CAD build for the part. Positions are in the model's coordinates, mm. Face numbers are marked on the shaded views. Give positions to 0.01 mm unless a question says otherwise; leave off trailing zeros. Use one line per item in the form item = value.
```python
from build123d import *

# Parameters (mm, degrees)
F0_W      = 40
F0_H      = 40
F1_DEPTH  = 10
F3_DEPTH  = 30
F4_R      = 5
F6_R      = 32.5
F7_DEPTH  = 5
F9_ANGLE  = -225
F10_ANGLE = -35.264


with BuildPart() as f1:
    # F0 (on Top) → F1 (new body)
    with BuildSketch(Plane.XY):
        with Locations((20, 20)):
            Rectangle(F0_W, F0_H)
    extrude(amount=F1_DEPTH)

    # F2 (on face) → F3 (join)
    with BuildSketch(Plane.XY.offset(10)):
        Polygon((0, 40), (0, 0), (40, 0), (40, 10), (10, 10), (10, 40), align=None)
    extrude(amount=F3_DEPTH)

    # F4
    f4_edges = [f1.edges().sort_by_distance(p)[0] for p in [
        (20, 0, 40),
        (0, 20, 40),
        (0, 0, 20),
        (20, 0, 0),
        (0, 20, 0),
        (20, 40, 0),
        (40, 20, 0),
        (40, 0, 20),
        (0, 40, 20),
    ]]
    fillet(f4_edges, radius=F4_R)

    # F6 (on 3pt) → F7 (cut)
    with BuildSketch(Plane(origin=(30, 30, 30), x_dir=(-0.8164965809, 0.4082482905, 0.4082482905), z_dir=(0.5773502692, 0.5773502692, 0.5773502692))):
        Circle(F6_R)
    extrude(amount=-F7_DEPTH, mode=Mode.SUBTRACT)


with BuildPart() as f1_1:
    # F9: moved
    add(f1.part.rotate(Axis((0, 27.5, 0), (0, 1, 0)), F9_ANGLE))


with BuildPart() as f1_2:
    # F10: moved
    add(f1_1.part.rotate(Axis((27.5, 0, 0), (1, 0, 0)), F10_ANGLE))


with BuildPart() as f1_3:
    # F13: moved
    add(f1_2.part.moved(Location((0, 0, 46.961))))


solid = f1_3.part
```
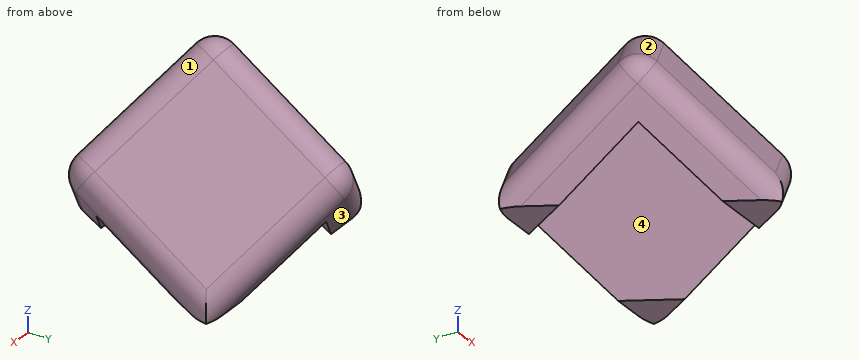
1. Drill centre lines: line 1 (Y direction, x = 8, z = 9.5); line 2 (X direction, y = 0, z = 4); line 3 (X direction, y = 11.5, z = 10.5). Where is each one in solid material? Low to high.
Result sheet:
line_1 = -25.52 to -14.24, 14.63 to 22.5
line_2 = -21.49 to -20.94, 20.94 to 21.49
line_3 = -23.13 to -8.99, 8.99 to 23.13
2. Mould opens along X. For the marked faces 1, 2, 3 and 4 say: pulls with the +X half, pulls with the -X half, needs draft (parallel to the pull), parting line crosses it, or undercut.
Result sheet:
face_1 = pulls with the +X half
face_2 = pulls with the -X half
face_3 = needs draft
face_4 = undercut
3. Drop flat-ended pins along their axis: P1, Ø1.5, axis at x = -4.5, y = -1.5, coming from the +Z side; P2, Ø1, axis at y = -4, z = 6.5, coming from the -X side; P3, Ø10, axis at y = -9.5, z = 5, coming from the +X side. Give the stop position or say it passes through.
Result sheet:
P1 = 41.58
P2 = -21.72
P3 = 21.82
